Print and shaded views of the part. All mm, measured from the part's lowest x, y and z. Round coordinates to 2 decimals unless told otherwise and drop trailing zeros. Write each loop counter-clockwise with the first axis right and the second up, starting at its lowest first coordinate (ties: lowest second). Pieces come first, ordered by that corner, then holes. Notation, with made-up numbers: (52, -36) -> (84, -36) arc R25 cw to (84, -6) -> close; hole circle Ø9 at (45.5, -2.5). An arc over 180 degrees is marked (long way). Use CSV: the item, a comma, the result in double quotes. Start each with the question number.
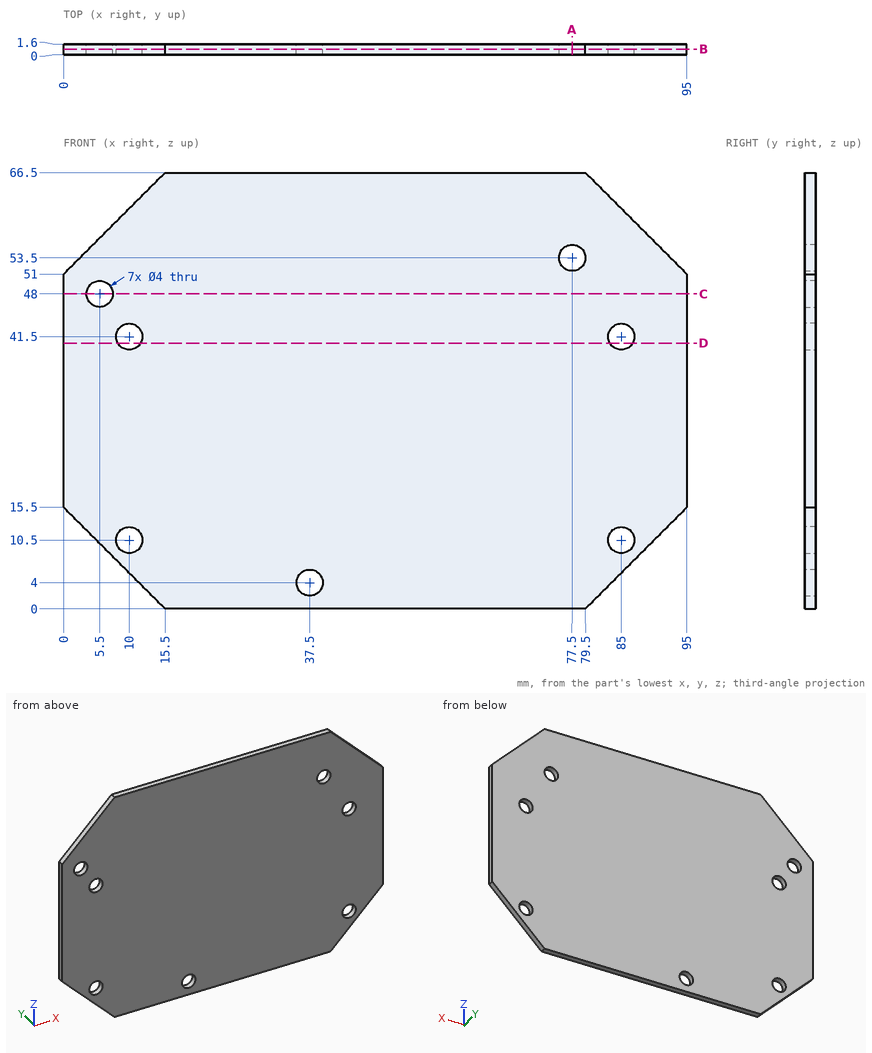
1. Band-saw the part on A-A (x = 77.5). List the corners of the cut face in (y, z).
2. Band-saw the part on D-D (z = 40.5). List the corners of the cut face in (x, y).
3. Band-saw the part on C-C (z = 48). List the corners of the cut face in (x, y), then the cut area to 3 significant figures.
4. Drill centre lines: line 1 along X through (y, z) = (0.95, 41.5); line 2 along Z through (x, y) = (84, 1.2); line 3 along X through (y, z) = (1, 4). Where is each one in solid material? Low to high. Write a range as [from, to].
5. Flat gauge pins, fed straight in: pin 1 (3 mm diameter, centred on x = 85, z = 10.5, fed in from -Y); pin 2 (5 mm diameter, centred on x = 85, z = 41.5, fed in from +Y). Where does each tip first touch, or does it go through?
6. Band-saw the part on B-B (y = 0.8). List the corners of the cut face in (x, z), then the cut area to 3 significant figures.
Answers below:
1,outline,"(0, 0) -> (1.6, 0) -> (1.6, 51.5) -> (0, 51.5) -> close; (0, 55.5) -> (1.6, 55.5) -> (1.6, 66.5) -> (0, 66.5) -> close"
2,outline,"(0, 0) -> (8.27, 0) -> (8.27, 1.6) -> (0, 1.6) -> close; (11.73, 0) -> (83.27, 0) -> (83.27, 1.6) -> (11.73, 1.6) -> close; (86.73, 0) -> (95, 0) -> (95, 1.6) -> (86.73, 1.6) -> close"
3,outline,"(0, 0) -> (3.5, 0) -> (3.5, 1.6) -> (0, 1.6) -> close; (7.5, 0) -> (95, 0) -> (95, 1.6) -> (7.5, 1.6) -> close"
3,area,"146 mm^2"
4,line 1,"x = [0, 8], [12, 83], [87, 95]"
4,line 2,"z = [4.5, 8.77], [12.23, 39.77], [43.23, 62]"
4,line 3,"x = [11.5, 35.5], [39.5, 83.5]"
5,pin 1,"passes through"
5,pin 2,"stops at y = 1.6"
6,outline,"(0, 15.5) -> (15.5, 0) -> (79.5, 0) -> (95, 15.5) -> (95, 51) -> (79.5, 66.5) -> (15.5, 66.5) -> (0, 51) -> close; hole circle Ø4 at (5.5, 48); hole circle Ø4 at (10, 10.5); hole circle Ø4 at (10, 41.5); hole circle Ø4 at (37.5, 4); hole circle Ø4 at (77.5, 53.5); hole circle Ø4 at (85, 10.5); hole circle Ø4 at (85, 41.5)"
6,area,"5,750 mm^2"
